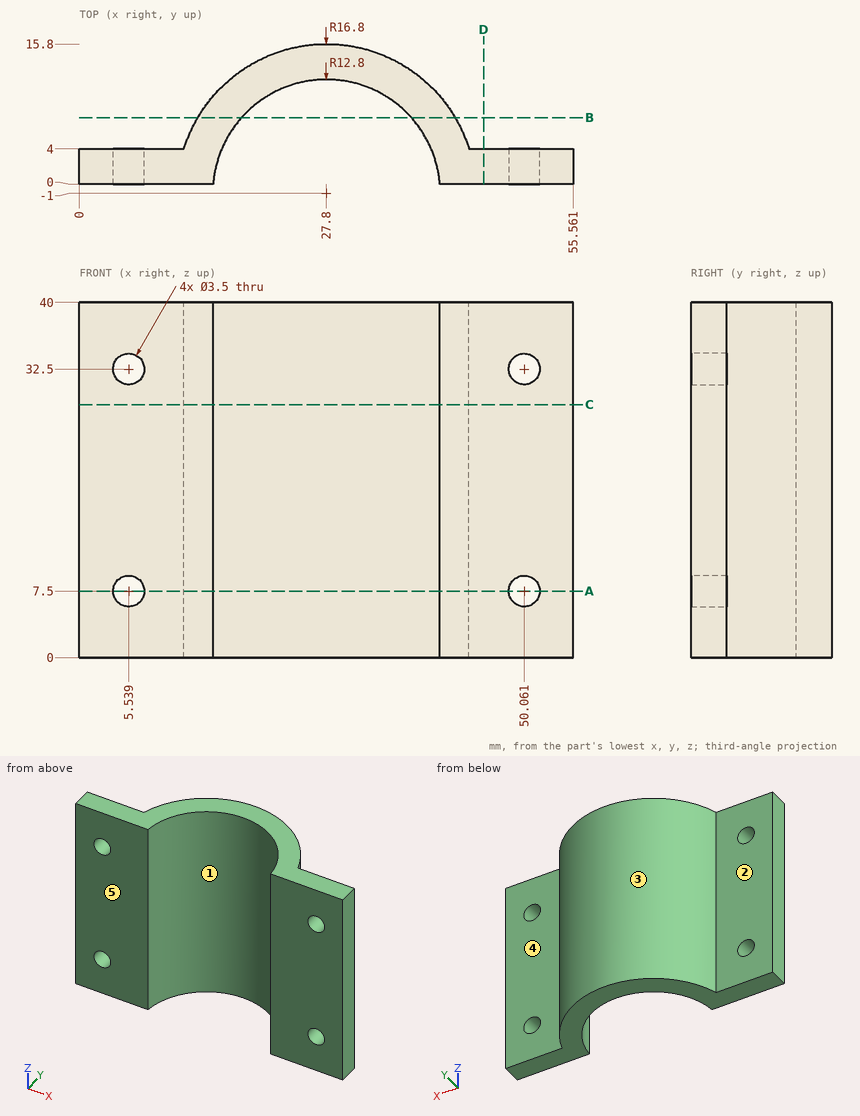
Input: dimensioned drawing with shaded views. Units: mm. Origin: part minimum x, y, z. A direction names the side the tool comes from. Coordinates: 2 decimals unless noted, no trailing zeros. Write each loop counter-clockwise with the first axis right and the second up, starting at its lowest first coordinate (ties: lowest second). Pieces come first, ordered by that corner, then holes. Notation, with made-up numbers: M 87,20.5 L 125,20.5 A8 cw 125,31.5 Z; hole C 8.25,22.5 d5. An arc over 180 degrees is marked long. Use a Markdown table: item, result.
1) Section B-B, the plane y = 7.5. Output: boundary loops of the cut face in (x, z), then the cut area to 3 significant figures.
Conclusion:
| item | result |
|---|---|
| outline | M 13.31,0 L 18.23,0 L 18.23,40 L 13.31,40 Z; M 37.37,0 L 42.29,0 L 42.29,40 L 37.37,40 Z |
| area | 394 mm^2 |
2) Mould query, pull axis X, two halves, no side actions, for the marked faces 1, 2 and 3. Classes: pulls with the +X half, pulls with the -X half, needs draft (parallel to the pull), parting line crosses it, or undercut.
Conclusion:
| item | result |
|---|---|
| face 1 | undercut |
| face 2 | needs draft |
| face 3 | parting line crosses it |
3) Section A-A, the plane z = 7.5. Output: boundary loops of the cut face in (x, y).
Conclusion:
| item | result |
|---|---|
| outline | M 0,0 L 3.79,0 L 3.79,4 L 0,4 Z; M 7.29,0 L 15.04,0 A12.8 cw 40.56,0 L 48.31,0 L 48.31,4 L 43.84,4 A16.8 ccw 11.76,4 L 7.29,4 Z; M 51.81,0 L 55.56,0 L 55.56,4 L 51.81,4 Z |
4) Section C-C, the plane z = 28.5. Output: boundary loops of the cut face in (x, y).
Conclusion:
| item | result |
|---|---|
| outline | M 0,0 L 15.04,0 A12.8 cw 40.56,0 L 55.56,0 L 55.56,4 L 43.84,4 A16.8 ccw 11.76,4 L 0,4 Z |
5) First-contact query: pin 1 Ø3 at (x, z) = (19, 26.5) entering from -Y; pin 2 Ø5 at (x, z) = (20.5, 22) entering from +Y; pin 3 Ø5 at (y, z) = (10, 14.5) entering from +X. Flat tips, straight axial feed; report the tip coordinate or a pass-through.
Conclusion:
| item | result |
|---|---|
| pin 1 | stops at y = 6.6 |
| pin 2 | stops at y = 15.1 |
| pin 3 | stops at x = 42.29 |
6) Reachability of the marked faces 4 and 5 from +Z, -Z, +X, -X, +Y, -Y: full face, straight path, thin tool, end or side. Return the list, or none.
Conclusion:
| item | result |
|---|---|
| face 4 | +Z, -Z, +X, +Y |
| face 5 | +Z, -Z, +X, -X, -Y |
7) Section D-D, the plane x = 45.5. Output: boundary loops of the cut face in (y, z).
Conclusion:
| item | result |
|---|---|
| outline | M 0,0 L 4,0 L 4,40 L 0,40 Z |
8) Ray query, L1, parallel to X at y = 7.75, z = 11; L2, parallel to Y at x = 52.5, z = 12.5; L3, parallel to Y at x = 14.5, z = 16.5. Return the intervals inside material, ascending.
Conclusion:
| item | result |
|---|---|
| L1 | x = 13.46 to 18.46, 37.14 to 42.14 |
| L2 | y = 0 to 4 |
| L3 | y = 0 to 9.26 |
